For this review, take the finished solid that the model builds, in its own axes (mm). A direction names the side the tool comes from. Coordinates: 2 decimals unless noted, no trailing zeros. Write each loop counter-clockwise with the first axis right and the second up, starting at its lowest first coordinate (ties: lowest second). Pieces come first, ordered by that corner, then holes. Notation, with made-up numbers: M 23,-3 L 30,-3 A38 ccw 30,36 Z; hole C -36.75,28.5 d4. An arc over 180 degrees is marked long. Return JSON: item names as keys, results as strings.
```python
from build123d import *

# Parameters (mm, degrees)
BOSS_EXTRUDE1_DEPTH = 60
SKETCH2_R           = 10
CUT_EXTRUDE1_DEPTH  = 60
CUT_EXTRUDE2_DEPTH  = 20
SKETCH6_R           = 10
CUT_EXTRUDE6_DEPTH  = 20
BOSS_EXTRUDE2_DEPTH = 20
BOSS_EXTRUDE3_DEPTH = 20
SKETCH9_W           = 40
SKETCH9_H           = 10
CUT_EXTRUDE7_DEPTH  = 95


with BuildPart() as part:
    # Sketch1 → Boss-Extrude1 (new body)
    with BuildSketch(Plane.XY):
        with BuildLine():
            ThreePointArc((-50, 0), (0, 50), (50, 0))
            Line((50, 0), (50, -50))
            Line((50, -50), (-50, -50))
            Line((-50, -50), (-50, 0))
        make_face()
    extrude(amount=BOSS_EXTRUDE1_DEPTH)

    # Sketch2 → Cut-Extrude1 (cut)
    with BuildSketch(Plane.XY.offset(60)):
        Circle(SKETCH2_R)
    extrude(amount=-CUT_EXTRUDE1_DEPTH, mode=Mode.SUBTRACT)

    # Sketch3 → Cut-Extrude2 (cut)
    with BuildSketch(Plane.XY.offset(60)):
        with BuildLine():
            Line((-20, 0), (-20, 45.82575695))
            ThreePointArc((-20, 45.82575695), (0, 50), (20, 45.82575695))
            Line((20, 45.82575695), (20, 0))
            ThreePointArc((20, 0), (0, -20), (-20, 0))
        make_face()
    extrude(amount=-CUT_EXTRUDE2_DEPTH, mode=Mode.SUBTRACT)

    # Sketch6 → Cut-Extrude6 (cut)
    with BuildSketch(Plane(origin=(0, 0, 0), x_dir=(-1, 0, 0), z_dir=(0, 0, -1))):
        with BuildLine():
            Line((-35, 35.707142143), (-35, 0))
            ThreePointArc((-35, 0), (0, -35), (35, 0))
            Line((35, 0), (35, 35.707142143))
            ThreePointArc((35, 35.707142143), (0, 50), (-35, 35.707142143))
        make_face()
        Circle(SKETCH6_R, mode=Mode.SUBTRACT)
    extrude(amount=-CUT_EXTRUDE6_DEPTH, mode=Mode.SUBTRACT)

    # Sketch7 → Boss-Extrude2 (add)
    with BuildSketch(Plane(origin=(0, 0, 0), x_dir=(-1, 0, 0), z_dir=(0, 0, -1))):
        with BuildLine():
            Line((-70, -50), (-50, -50))
            Line((-50, -50), (-50, 0))
            ThreePointArc((-50, 0), (-46.097722286, 19.364916731), (-35, 35.707142143))
            Line((-35, 35.707142143), (-35, 60.621778265))
            ThreePointArc((-35, 60.621778265), (-60.621778265, 35), (-70, 0))
            Line((-70, 0), (-70, -50))
        make_face()
        with BuildLine():
            Line((-50, -50), (-35, -50))
            Line((-35, -50), (-35, 0))
            Line((-35, 0), (-35, 35.707142143))
            ThreePointArc((-35, 35.707142143), (-46.097722286, 19.364916731), (-50, 0))
            Line((-50, 0), (-50, -50))
        make_face()
        with BuildLine():
            ThreePointArc((50, 0), (46.097722286, 19.364916731), (35, 35.707142143))
            Line((35, 35.707142143), (35, 0))
            Line((35, 0), (35, -50))
            Line((35, -50), (50, -50))
            Line((50, -50), (50, 0))
        make_face()
        with BuildLine():
            ThreePointArc((70, 0), (60.621778265, 35), (35, 60.621778265))
            Line((35, 60.621778265), (35, 35.707142143))
            ThreePointArc((35, 35.707142143), (46.097722286, 19.364916731), (50, 0))
            Line((50, 0), (50, -50))
            Line((50, -50), (70, -50))
            Line((70, -50), (70, 0))
        make_face()
    extrude(amount=BOSS_EXTRUDE2_DEPTH)

    # Sketch8 → Boss-Extrude3 (add)
    with BuildSketch(Plane(origin=(0, 0, 0), x_dir=(-1, 0, 0), z_dir=(0, 0, -1))):
        with BuildLine():
            Line((-35, -50), (35, -50))
            Line((35, -50), (35, 0))
            ThreePointArc((35, 0), (0, -35), (-35, 0))
            Line((-35, 0), (-35, -50))
        make_face()
    extrude(amount=BOSS_EXTRUDE3_DEPTH)

    # Sketch9 → Cut-Extrude7 (cut)
    with BuildSketch(Plane.XZ.offset(50)):
        with Locations((0, -15)):
            Rectangle(SKETCH9_W, SKETCH9_H)
    extrude(amount=-CUT_EXTRUDE7_DEPTH, mode=Mode.SUBTRACT)


solid = part.part
```
1. We need section C-C (y = 42.5). State the section outline as (x, z) points, plus the area to 3 significant figures.
Checks:
{"outline": "M -55.62,-20 L -35,-20 L -35,0 L -55.62,0 Z; M -26.34,20 L 26.34,20 L 26.34,60 L 20,60 L 20,40 L -20,40 L -20,60 L -26.34,60 Z; M 35,-20 L 55.62,-20 L 55.62,0 L 35,0 Z", "area": "2,130 mm2"}
2. Draft analysis for pull direction X (two halves, no side actions). For faces 6 (the face through (60.364, 35.443, -9.86)), 7 (the face through (-35, 24, -4)), 8 (the face through (-56, 6, 0)), state which applies: +X half, -X half, draft (parallel to the pull), parting line (faces both ways), or undercut.
Checks:
{"face 6": "+X half", "face 7": "undercut", "face 8": "draft"}
3. We need section D-D (z = -7). State the section outline as (x, y) points, plus the area to 3 significant figures.
Checks:
{"outline": "M -70,-50 L 70,-50 L 70,0 A70 ccw 35,60.62 L 35,0 A35 cw -35,0 L -35,60.62 A70 ccw -70,0 Z", "area": "8,090 mm2"}
4. Clearance check with flat-ended pins moving along their axes: pin 1 Ø2 at (y, z) = (3.5, 9) entering from -X; pin 2 Ø6.5 at (x, y) = (6, -39) entering from -Z; pin 3 Ø22 at (y, z) = (12, 47.5) entering from +X; pin 4 Ø10 at (x, z) = (-50.5, 33) entering from -Y. State where each tip first meets the part, or that it passes through.
Checks:
{"pin 1": "x = -49.94", "pin 2": "z = -10", "pin 3": "x = 49.99", "pin 4": "y = -50"}
5. We need section A-A (x = 0). State the section outline as (y, z) points, plus the area to 3 significant figures.
Checks:
{"outline": "M -50,-10 L -35,-10 L -35,20 L -10,20 L -10,40 L -20,40 L -20,60 L -50,60 Z; M 10,20 L 50,20 L 50,40 L 10,40 Z", "area": "2,650 mm2"}
6. We need section B-B (z = 31.5). State the section outline as (x, y) points.
Checks:
{"outline": "M -50,-50 L 50,-50 L 50,0 A50 ccw -50,0 Z; hole C 0,0 d20"}
7. For faces 1 (the face through (-50, -25, 30)), 2 (the face through (8, 8, 20)), 3 (the face through (0, 23, 40)), 4 (the face through (50, -25, 30)), 5 (the face through (20, -40, -15)), list the 3-axis set-ups (+Z, -Z, +X, -X, +Y, -Y) from which the entire face can be reached by the end or side of a thin tool; tool diameter is ignored.
Checks:
{"face 1": "+Z, -X, +Y, -Y", "face 2": "-Z, +Y", "face 3": "+Z, +Y", "face 4": "+Z, +X, +Y, -Y", "face 5": "-Z, +Y, -Y"}
8. Wall thickness on L1, parallel to Y at x = 0, z = 35.5; L2, parallel to X at y = -42, z = -14.5; L3, parallel to Z at x = 40.5, y = 52: over which ranges is each line inside the solid? List them lowest first. Write a range as from..to.
Checks:
{"L1": "-50..-10, 10..50", "L2": "-70..-20, 20..70", "L3": "-20..0"}
